from build123d import *

# Parameters (mm, degrees)
CROQUIS1_R              = 10
SALIENTE_EXTRUIR1_DEPTH = 3
CROQUIS2_R              = 0.75
CROQUIS4_R              = 7.5
CORTAR_EXTRUIR1_DEPTH   = 15.456832295


with BuildPart() as part:
    # Croquis1 → Saliente-Extruir1 (new body)
    with BuildSketch(Plane(origin=(0, 0, 0), x_dir=(1, 0, 0), z_dir=(0, 1, 0))):
        with Locations(Location((0, 0, 0), (0, 0, 270))):
            Circle(CROQUIS1_R)
    extrude(amount=SALIENTE_EXTRUIR1_DEPTH)

    # Croquis2 → Cortar-Revolución1 (revolve, cut)
    with BuildSketch(Plane(origin=(0, 0, 0), x_dir=(0, 0, -1), z_dir=(1, 0, 0)), mode=Mode.PRIVATE) as cortar_revoluci_n1_sk:
        with Locations((10, 1.5)):
            Circle(CROQUIS2_R)
    revolve(cortar_revoluci_n1_sk.sketch.rotate(Axis((0, 3, 0), (0, -1, 0)), 180), axis=Axis((0, 3, 0), (0, -1, 0)), mode=Mode.SUBTRACT)

    # Croquis4 → Cortar-Extruir1 (cut, through all)
    with BuildSketch(Plane.XZ):
        with Locations(Location((0, 0, 0), (0, 0, 270))):
            Circle(CROQUIS4_R)
    extrude(amount=-CORTAR_EXTRUIR1_DEPTH, mode=Mode.SUBTRACT)


solid = part.part
Can you work these out from the model? Positions are in its coordinate system, mm. Coordinates: 2 decimals unless noted, no trailing zeros. Loops run counter-clockwise (first coordinate to the right, second up) from the corner with the lowest first, then second, coordinate; pieces in that order, holes last. Notation, with made-up numbers: (-22.75, 82) - (9.25, 82) arc R29 ccw to (9.25, 105) - close; hole circle Ø11 at (74.25, -7.75). An arc over 180 degrees is marked (long way). Answer as a JSON object with one key per item and string values. Group by question number.
Item 1: If we mould it in two halves opening along X, with no side actions, what happens to faces 1 (the face through (0.33, 1.479, 7.493)), 2 (the face through (-9.76, 2.62, -2.17)), 3 (the face through (7, 3, 4))? For each: released by +X, released by -X, zero draft, split by the parting line, or undercut.
Item 2: If we section it at B-B (z = 0): List the corners of the cut face in (x, y) for me.
Item 3: If we section it at C-C (y = 1.65): List the corners of the cut face in (x, z) for me.
Item 4: For pin 1 (1 mm diameter, centred on y = 2, z = -6.5, fed in from +X); pin 2 (1.5 mm diameter, centred on y = 1, z = 6, fed in from +X), each with a flat end and sliding along its axis, tell me the tip position at first contact or that it passes through.
Item 5: If I drill on L1, parallel to Z at x = -1.25, y = 0.35; L2, parallel to X at y = 2.05, z = 0; L3, parallel to X at y = 0.2, z = -1.75, over which ranges is the centre line in solid material (lowest first)? Write a range as from..to.
Item 6: If we section it at A-A (x = 0): List the corners of the cut face in (y, z) for me, plus the area to 3 significant figures.
Returned:
{
 "1": {"face 1": "undercut", "face 2": "split by the parting line", "face 3": "zero draft"},
 "2": {"outline": "(-10, 0) - (-7.5, 0) - (-7.5, 3) - (-10, 3) - (-10, 2.25) arc R0.75 cw to (-10, 0.75) - close; (7.5, 0) - (10, 0) - (10, 0.75) arc R0.75 cw to (10, 2.25) - (10, 3) - (7.5, 3) - close"},
 "3": {"outline": "circle Ø18.53 at (0, 0); hole circle Ø15 at (0, 0)"},
 "4": {"pin 1": "stops at x = 7.95", "pin 2": "stops at x = 8.48"},
 "5": {"L1": "z = -9.92..-7.4, 7.4..9.92", "L2": "x = -9.49..-7.5, 7.5..9.49", "L3": "x = -9.85..-7.29, 7.29..9.85"},
 "6": {"outline": "(0, -10) - (0.75, -10) arc R0.75 cw to (2.25, -10) - (3, -10) - (3, -7.5) - (0, -7.5) - close; (0, 7.5) - (3, 7.5) - (3, 10) - (2.25, 10) arc R0.75 cw to (0.75, 10) - (0, 10) - close", "area": "13.2 mm²"}
}
